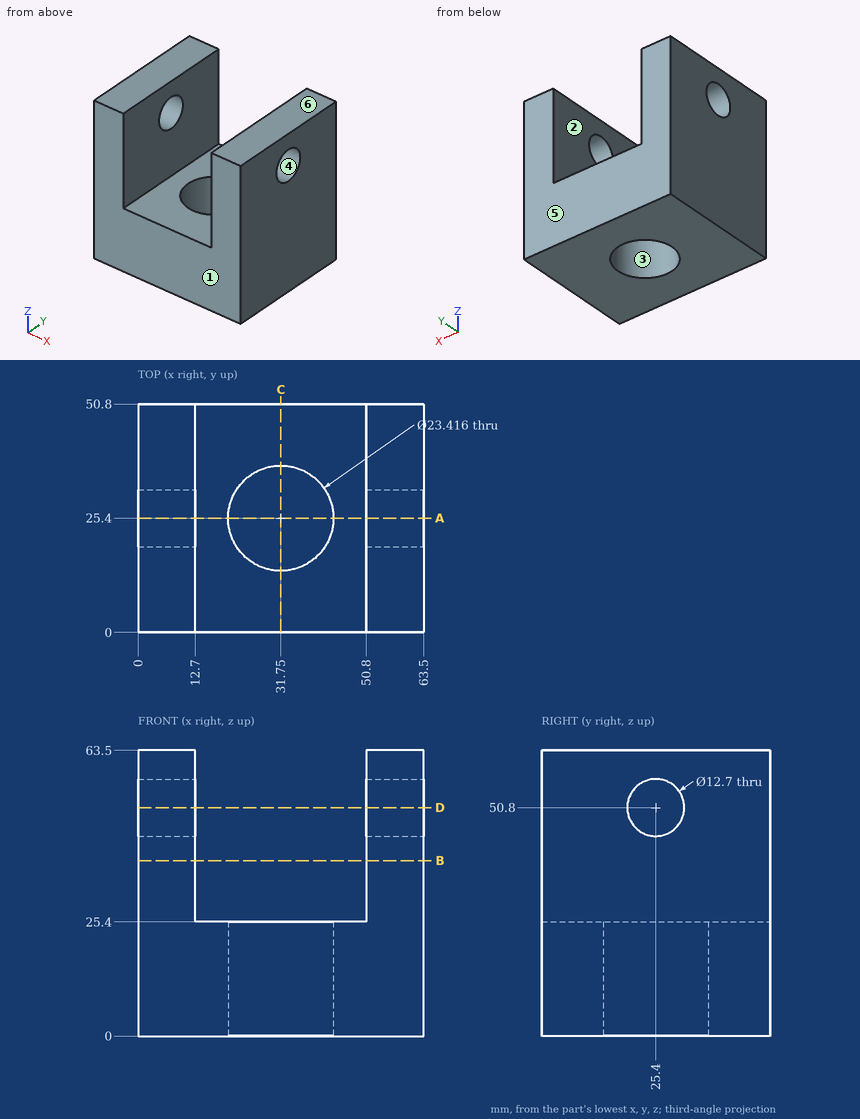
Input: dimensioned drawing with shaded views. Units: mm. Origin: part minimum x, y, z. A direction names the side the tool comes from. Round coordinates to 2 decimals unless told otherwise and drop trailing zeros. Order: outer loops, then holes, each group sorted by start corner. A loop starts at its lowest first (then second) coordinate and runs counter-clockwise, first axis right, second up. Notation, with made-up numbers: (19.25, 85) - (60.25, 85) arc R25 ccw to (60.25, 122) - close; hole circle Ø2 at (-15.75, 3.25). An arc over 180 degrees is marked (long way). Write item = value, one per line. Start each with the question number.
Q1. Cut plane D-D on z = 50.8. Return the cut outline in (x, y).
Q2. Cut plane B-B on z = 39. Return the cut outline in (x, y).
Q3. Ray query, line 1 (Y direction, x = 31.75, z = 14); line 2 (Z direction, x = 3, y = 25); line 3 (X direction, y = 31, z = 44.5). Return the intervals inside material, ascending. Write a range as from..to.
Q4. Cut plane C-C on x = 31.75. Return the cut outline in (y, z).
Q5. Pin query (flat end, axial travel): pin 1 (11.5 mm diameter, centred on x = 24.5, y = 19.5, fed in from +Z). Return the tip coordinate at first contact, or that it passes through.
Q6. Cut plane A-A on y = 25.4. Return the cut outline in (x, z).
Q7. Access query for the marked faces 1 and 2. Directions: +Z, -Z, +X, -X, +Y, -Y. A direction counts if a zero-diameter tool reaches every point of the face in a straight line with its end or side. Return the directions, or none.
Q8. Pull-direction query (Y, two-part tool) for the marked faces 3, 4, 5 and 6; classes: +Y half, -Y half, draft (parallel to the pull), parting line (faces both ways), or undercut.
Outcome:
q1.outline = (0, 0) - (12.7, 0) - (12.7, 19.05) - (0, 19.05) - close; (0, 31.75) - (12.7, 31.75) - (12.7, 50.8) - (0, 50.8) - close; (50.8, 0) - (63.5, 0) - (63.5, 19.05) - (50.8, 19.05) - close; (50.8, 31.75) - (63.5, 31.75) - (63.5, 50.8) - (50.8, 50.8) - close
q2.outline = (0, 0) - (12.7, 0) - (12.7, 50.8) - (0, 50.8) - close; (50.8, 0) - (63.5, 0) - (63.5, 50.8) - (50.8, 50.8) - close
q3.line_1 = 0..13.69, 37.11..50.8
q3.line_2 = 0..44.46, 57.14..63.5
q3.line_3 = 0..12.7, 50.8..63.5
q4.outline = (0, 0) - (13.69, 0) - (13.69, 25.4) - (0, 25.4) - close; (37.11, 0) - (50.8, 0) - (50.8, 25.4) - (37.11, 25.4) - close
q5.pin_1 = 25.4
q6.outline = (0, 0) - (20.04, 0) - (20.04, 25.4) - (12.7, 25.4) - (12.7, 44.45) - (0, 44.45) - close; (0, 57.15) - (12.7, 57.15) - (12.7, 63.5) - (0, 63.5) - close; (43.46, 0) - (63.5, 0) - (63.5, 44.45) - (50.8, 44.45) - (50.8, 25.4) - (43.46, 25.4) - close; (50.8, 57.15) - (63.5, 57.15) - (63.5, 63.5) - (50.8, 63.5) - close
q7.face_1 = +Z, -Z, +X, -X, -Y
q7.face_2 = +Z, +Y, -Y
q8.face_3 = undercut
q8.face_4 = undercut
q8.face_5 = +Y half
q8.face_6 = draft
